from build123d import *

# Parameters (mm, degrees)
SKETCH2_R           = 31.75
BOSS_EXTRUDE1_DEPTH = 6.35
BOSS_EXTRUDE2_DEPTH = 6.35
SKETCH4_R           = 3.3782
CUT_EXTRUDE1_DEPTH  = 47.6627796
FILLET2_R           = 0.79375
SKETCH5_R           = 2.159
CUT_EXTRUDE2_DEPTH  = 47.6627796
FILLET3_R           = 1.5875


with BuildPart() as part:
    # Sketch2 → Boss-Extrude1 (new body)
    with BuildSketch(Plane.XY):
        Circle(SKETCH2_R)
    extrude(amount=BOSS_EXTRUDE1_DEPTH)

    # Sketch3 → Boss-Extrude2 (add)
    with BuildSketch(Plane.XY.offset(6.35)):
        with BuildLine():
            Line((3.937, 30.411026388), (3.937, 20.6375))
            ThreePointArc((3.937, 20.6375), (0, 16.7005), (-3.937, 20.6375))
            Line((-3.937, 20.6375), (-3.937, 30.411026388))
            ThreePointArc((-3.937, 30.411026388), (-12.7, 21.997045256), (-24.368221407, 18.615055209))
            Line((-24.368221407, 18.615055209), (-15.904099271, 13.728292015))
            ThreePointArc((-15.904099271, 13.728292015), (-14.463057256, 8.35025), (-19.841099271, 6.909207985))
            Line((-19.841099271, 6.909207985), (-28.305221407, 11.795971179))
            ThreePointArc((-28.305221407, 11.795971179), (-25.4, 0), (-28.305221407, -11.795971179))
            Line((-28.305221407, -11.795971179), (-19.841099271, -6.909207985))
            ThreePointArc((-19.841099271, -6.909207985), (-14.463057256, -8.35025), (-15.904099271, -13.728292015))
            Line((-15.904099271, -13.728292015), (-24.368221407, -18.615055209))
            ThreePointArc((-24.368221407, -18.615055209), (-12.7, -21.997045256), (-3.937, -30.411026388))
            Line((-3.937, -30.411026388), (-3.937, -20.6375))
            ThreePointArc((-3.937, -20.6375), (0, -16.7005), (3.937, -20.6375))
            Line((3.937, -20.6375), (3.937, -30.411026388))
            ThreePointArc((3.937, -30.411026388), (12.7, -21.997045256), (24.368221407, -18.615055209))
            Line((24.368221407, -18.615055209), (15.904099271, -13.728292015))
            ThreePointArc((15.904099271, -13.728292015), (14.463057256, -8.35025), (19.841099271, -6.909207985))
            Line((19.841099271, -6.909207985), (28.305221407, -11.795971179))
            ThreePointArc((28.305221407, -11.795971179), (25.4, 0), (28.305221407, 11.795971179))
            Line((28.305221407, 11.795971179), (19.841099271, 6.909207985))
            ThreePointArc((19.841099271, 6.909207985), (14.463057256, 8.35025), (15.904099271, 13.728292015))
            Line((15.904099271, 13.728292015), (24.368221407, 18.615055209))
            ThreePointArc((24.368221407, 18.615055209), (12.7, 21.997045256), (3.937, 30.411026388))
        make_face()
    extrude(amount=BOSS_EXTRUDE2_DEPTH)

    # Sketch4 → Cut-Extrude1 (cut, through all)
    with BuildSketch(Plane.XY.offset(12.7)):
        Circle(SKETCH4_R)
    extrude(amount=-CUT_EXTRUDE1_DEPTH, mode=Mode.SUBTRACT)

    # Fillet2
    fillet2_edges = [part.edges().sort_by_distance(p)[0] for p in [
        (-28.305221407, 11.795971179, 9.525),
        (-28.305221407, -11.795971179, 9.525),
        (-24.368221407, -18.615055209, 9.525),
        (-3.937, -30.411026388, 9.525),
        (3.937, -30.411026388, 9.525),
        (24.368221407, -18.615055209, 9.525),
        (28.305221407, -11.795971179, 9.525),
        (28.305221407, 11.795971179, 9.525),
        (24.368221407, 18.615055209, 9.525),
        (3.937, 30.411026388, 9.525),
        (-3.937, 30.411026388, 9.525),
        (-24.368221407, 18.615055209, 9.525),
    ]]
    fillet(fillet2_edges, radius=FILLET2_R)

    # Sketch5 → Cut-Extrude2 (cut, through all)
    with BuildSketch(Plane(origin=(0, 0, 0), x_dir=(-1, 0, 0), z_dir=(0, 0, -1))):
        with Locations((-11.90625, 20.622229928)):
            Circle(SKETCH5_R)
        with Locations((11.90625, 20.622229928)):
            Circle(SKETCH5_R)
        with Locations((23.8125, 0)):
            Circle(SKETCH5_R)
        with Locations((11.90625, -20.622229928)):
            Circle(SKETCH5_R)
        with Locations((-11.90625, -20.622229928)):
            Circle(SKETCH5_R)
        with Locations((-23.8125, 0)):
            Circle(SKETCH5_R)
    extrude(amount=-CUT_EXTRUDE2_DEPTH, mode=Mode.SUBTRACT)

    # Fillet3
    # the kernel refuses this fillet: 1.5875 mm, written as the material it takes off along each edge
    with BuildSketch(Plane(origin=(25.439668824, 1.419014665, 17.971488678), x_dir=(-0.895364972347459, 0.44533309588804865, 0), z_dir=(0, 0, -1)), Plane(origin=(13.94873716, -21.321892132, 17.971488678), x_dir=(-0.062012711988979966, 0.9980753596556584, 0), z_dir=(0, 0, -1)), Plane(origin=(-11.490931663, -22.740906798, 17.971488678), x_dir=(0.8333522603583425, 0.5527422637682424, 0), z_dir=(0, 0, -1)), Plane(origin=(-25.439668824, -1.419014665, 17.971488678), x_dir=(0.895364972347876, -0.44533309588721026, 0), z_dir=(0, 0, -1)), Plane(origin=(-13.94873716, 21.321892132, 17.971488678), x_dir=(0.06201271198937459, -0.998075359655634, 0), z_dir=(0, 0, -1)), Plane(origin=(11.490931663, 22.740906798, 17.971488678), x_dir=(-0.8333522603586354, -0.552742263767801, 0), z_dir=(0, 0, -1))) as fillet3_piece_1:
        with BuildLine():
            CenterArc((2.256551384, 1.467035409), FILLET3_R, 161.515751163, 86.019798363)
            ThreePointArc((0.75094916, 1.970342665), (0.395929534, 0.977375414), (0, 0))
            ThreePointArc((0, 0), (0.824975775, 0.163831844), (1.64995155, 0))
        make_face()
    extrude(amount=11.621488678, mode=Mode.SUBTRACT)
    with BuildSketch(Plane(origin=(25.439668824, -1.419014665, 17.971488678), x_dir=(0.09726153154123053, -0.9952588580275255, 0), z_dir=(0, 0, -1)), Plane(origin=(11.490931663, -22.740906798, 17.971488678), x_dir=(-0.8132886886226861, -0.581860386139486, 0), z_dir=(0, 0, -1)), Plane(origin=(-13.94873716, -21.321892132, 17.971488678), x_dir=(-0.9105502201639705, 0.4133984718880138, 0), z_dir=(0, 0, -1)), Plane(origin=(-25.439668824, 1.419014665, 17.971488678), x_dir=(-0.09726153154127945, 0.9952588580275207, 0), z_dir=(0, 0, -1)), Plane(origin=(-11.490931663, 22.740906798, 17.971488678), x_dir=(0.8132886886227111, 0.5818603861394509, 0), z_dir=(0, 0, -1)), Plane(origin=(13.94873716, 21.321892132, 17.971488678), x_dir=(0.9105502201639343, -0.41339847188809375, 0), z_dir=(0, 0, -1))) as fillet3_piece_2:
        with BuildLine():
            CenterArc((2.17448908, 1.586131862), FILLET3_R, 181.601297313, 86.019798363)
            ThreePointArc((0.587609026, 1.541770329), (0.446894509, 0.71253856), (0, 0))
            ThreePointArc((0, 0), (1.054297736, 0.021890215), (2.108595471, 0))
        make_face()
    extrude(amount=11.621488678, mode=Mode.SUBTRACT)


solid = part.part
CAD build for the part. Positions are in the model's coordinates, mm. A direction names the side the tool comes from. Coordinates: 2 decimals unless noted, no trailing zeros. Order: outer loops, then holes, each group sorted by start corner. A loop starts at its lowest first (then second) coordinate and runs counter-clockwise, first axis right, second up. Notation, with made-up numbers: (17.25, -36) -> (63.25, -36) arc R16 cw to (63.25, -23) -> close; hole circle Ø11 at (80.5, 73.25). An arc over 180 degrees is marked (long way). Answer in a Markdown table with one row per item.
1) Band-saw the part on B-B (y = 0). List the corners of the cut face in (x, z).
Check values:
| item | result |
|---|---|
| outline | (-31.75, 0) -> (-25.97, 0) -> (-25.97, 6.35) -> (-31.75, 6.35) -> close; (-21.65, 0) -> (-3.38, 0) -> (-3.38, 12.7) -> (-21.65, 12.7) -> close; (3.38, 0) -> (21.65, 0) -> (21.65, 12.7) -> (3.38, 12.7) -> close; (25.97, 0) -> (31.75, 0) -> (31.75, 6.35) -> (25.97, 6.35) -> close |
2) Mould opens along Y. For faces 4 (the face through (14.689, 20.455, 9.569)), 5 (the face through (0, -7, 0)), 6 (the face through (-2.681, -2.056, 6.439)) say: pulls with the +Y half, pulls with the -Y half, needs draft (parallel to the pull), parting line crosses it, or undercut.
Check values:
| item | result |
|---|---|
| face 4 | pulls with the +Y half |
| face 5 | needs draft |
| face 6 | undercut |
3) Which spindle directions (+Z, -Z, +X, -X, +Y, -Y) get a long thin tool onto all of the face, cutting with end or side? Do faces 1 (the face through (-7.399, 26.074, 9.481)), 2 (the face through (-22.58, -18.19, 9.57)), 3 (the face through (0.1, 16.7, 9.5)). Say none if no direction does.
Check values:
| item | result |
|---|---|
| face 1 | +Z, -X, +Y |
| face 2 | +Z, -X |
| face 3 | +Z, +Y |
4) Band-saw the part on D-D (x = -7.5). List the corners of the cut face in (y, z), and give its area (3 significant figures).
Check values:
| item | result |
|---|---|
| outline | (-30.85, 0) -> (30.85, 0) -> (30.85, 6.35) -> (25.97, 6.35) -> (25.97, 12.7) -> (-25.97, 12.7) -> (-25.97, 6.35) -> (-30.85, 6.35) -> close |
| area | 722 mm2 |
5) Band-saw the part on C-C (z = 1.25). List the corners of the cut face in (x, y), and give its area (3 significant figures).
Check values:
| item | result |
|---|---|
| outline | circle Ø63.5 at (0, 0); hole circle Ø4.32 at (-23.81, 0); hole circle Ø4.32 at (-11.91, -20.62); hole circle Ø4.32 at (-11.91, 20.62); hole circle Ø6.76 at (0, 0); hole circle Ø4.32 at (11.91, -20.62); hole circle Ø4.32 at (11.91, 20.62); hole circle Ø4.32 at (23.81, 0) |
| area | 3,040 mm2 |
6) Drill centre lines: line 1 (X direction, y = -22.5, z = 10.5); line 2 (Y direction, x = 0, z = 3.5); line 3 (Y direction, x = 16.5, z = 10.5). Where is each one in solid material? Low to high.
Check values:
| item | result |
|---|---|
| line 1 | -10.37 to -3.94, 3.94 to 10.37 |
| line 2 | -31.75 to -3.38, 3.38 to 31.75 |
| line 3 | -20.2 to -14.07, -6.63 to 6.63, 14.07 to 20.2 |
7) Flat gauge pins, fed straight in: P1, Ø2, axis at x = 18.5, y = -18, coming from the -Z side; P2, Ø3, axis at y = 24.5, z = 9.5, coming from the -X side; P3, Ø7, axis at y = 25.5, z = 10, coming from the +X side; P4, Ø3, axis at x = -4, z = 11, coming from the -Y side. Where does each tip first touch, or does it go through?
Check values:
| item | result |
|---|---|
| P1 | z = 0 |
| P2 | x = -10.36 |
| P3 | x = 10.39 |
| P4 | y = -28.7 |
8) Band-saw the part on A-A (x = 0). List the corners of the cut face in (y, z), and give its area (3 significant figures).
Check values:
| item | result |
|---|---|
| outline | (-31.75, 0) -> (-3.38, 0) -> (-3.38, 12.7) -> (-16.7, 12.7) -> (-16.7, 6.35) -> (-31.75, 6.35) -> close; (3.38, 0) -> (31.75, 0) -> (31.75, 6.35) -> (16.7, 6.35) -> (16.7, 12.7) -> (3.38, 12.7) -> close |
| area | 530 mm2 |
